Work out the finished part from the listing and answer in its coordinate system (mm). Coordinates: 2 decimals unless noted, no trailing zeros. Loops run counter-clockwise (first coordinate to the right, second up) from the corner with the lowest first, then second, coordinate; pieces in that order, holes last. Notation, with made-up numbers: (37.5, 20) -> (52.5, 20) arc R21 cw to (52.5, 40) -> close; hole circle Ø3 at (62.5, 77). An arc over 180 degrees is marked (long way). Use a Markdown table: item, result. Add a question column.
```python
from build123d import *

# Parameters (mm, degrees)
SKETCH1_R           = 3.175
BOSS_EXTRUDE1_DEPTH = 12.7
SKETCH3_R           = 3.175
CUT_EXTRUDE1_DEPTH  = 117.653215918


with BuildPart() as part:
    # Sketch1 → Boss-Extrude1 (new body)
    with BuildSketch(Plane(origin=(0, 0, 0), x_dir=(1, 0, 0), z_dir=(0, 1, 0))):
        Polygon((0, 97.028), (63.5, 97.028), (63.5, 0), (-63.5, 0), (-63.5, 97.028), align=None)
        with Locations(Location((-42.926, 48.514, 0), (0, 0, 270))):
            Circle(SKETCH1_R, mode=Mode.SUBTRACT)
        with Locations(Location((42.926, 48.514, 0), (0, 0, 270))):
            Circle(SKETCH1_R, mode=Mode.SUBTRACT)
    extrude(amount=BOSS_EXTRUDE1_DEPTH)

    # Sketch3 → Cut-Extrude1 (cut, through all)
    with BuildSketch(Plane.XY):
        with Locations((-31.75, 6.35)):
            Circle(SKETCH3_R)
        with Locations((31.75, 6.35)):
            Circle(SKETCH3_R)
    extrude(amount=-CUT_EXTRUDE1_DEPTH, mode=Mode.SUBTRACT)


solid = part.part
```
Item 1: Section C-C (z = -19) is taken. Determine the outline of the cut face in (x, y) (3 decimals), then the cut area to 3 significant figures.
Item 2: Find the intervals of material crossed by probe 1 along Y at (x, z) = (31.75, -29) (3 decimals); probe 2 along X at (y, z) = (8.5, -76); probe 3 along X at (y, z) = (12, -48), in increasing order.
Item 3: Section B-B (x = 31.75) is taken. Determine the outline of the cut face in (y, z) (3 decimals).
Item 4: Section A-A (y = 6.35) is taken. Determine the outline of the cut face in (x, z) (3 decimals).
Item 5: For a pull along X with two mould halves and no side action, classify faces 1 (the face through (1, 12.7, -49)), 2 (the face through (63.5, 6, -49)), 3 (the face through (33.5, 9, -47.8)), 4 (the face through (-42.786, 6.261, -51.686)) as +X half, -X half, draft (parallel to the pull), parting line (faces both ways), or undercut.
Output:
| question | item | result |
|---|---|---|
| 1 | outline | (-63.5, 0) -> (63.5, 0) -> (63.5, 12.7) -> (-63.5, 12.7) -> close; hole circle Ø6.35 at (-31.75, 6.35); hole circle Ø6.35 at (31.75, 6.35) |
| 1 | area | 1,550 mm2 |
| 2 | probe 1 | y = 0 to 3.175, 9.525 to 12.7 |
| 2 | probe 2 | x = -63.5 to -34.09, -29.41 to 29.41, 34.09 to 63.5 |
| 2 | probe 3 | x = -63.5 to -46.06, -39.79 to 39.79, 46.06 to 63.5 |
| 3 | outline | (0, -97.028) -> (3.175, -97.028) -> (3.175, 0) -> (0, 0) -> close; (9.525, -97.028) -> (12.7, -97.028) -> (12.7, 0) -> (9.525, 0) -> close |
| 4 | outline | (-63.5, -97.028) -> (-34.925, -97.028) -> (-34.925, 0) -> (-63.5, 0) -> close; (-28.575, -97.028) -> (28.575, -97.028) -> (28.575, 0) -> (-28.575, 0) -> close; (34.925, -97.028) -> (63.5, -97.028) -> (63.5, 0) -> (34.925, 0) -> close; hole circle Ø6.35 at (-42.926, -48.514); hole circle Ø6.35 at (42.926, -48.514) |
| 5 | face 1 | draft |
| 5 | face 2 | +X half |
| 5 | face 3 | undercut |
| 5 | face 4 | undercut |
